Check sheet for the drawn part. Datum: minimum x, y, z corner. Units: mm. Round coordinates to 2 decimals unless told otherwise and drop trailing zeros. Write each loop counter-clockwise with the first axis right and the second up, starting at its lowest first coordinate (ties: lowest second). Pieces come first, ordered by that corner, then holes. Notation, with made-up numbers: (70.5, -4) -> (86.5, -4) arc R6 ccw to (86.5, 6) -> close; hole circle Ø10 at (67, 76.25). An arc over 180 degrees is marked (long way). Use a Markdown table: item, result.
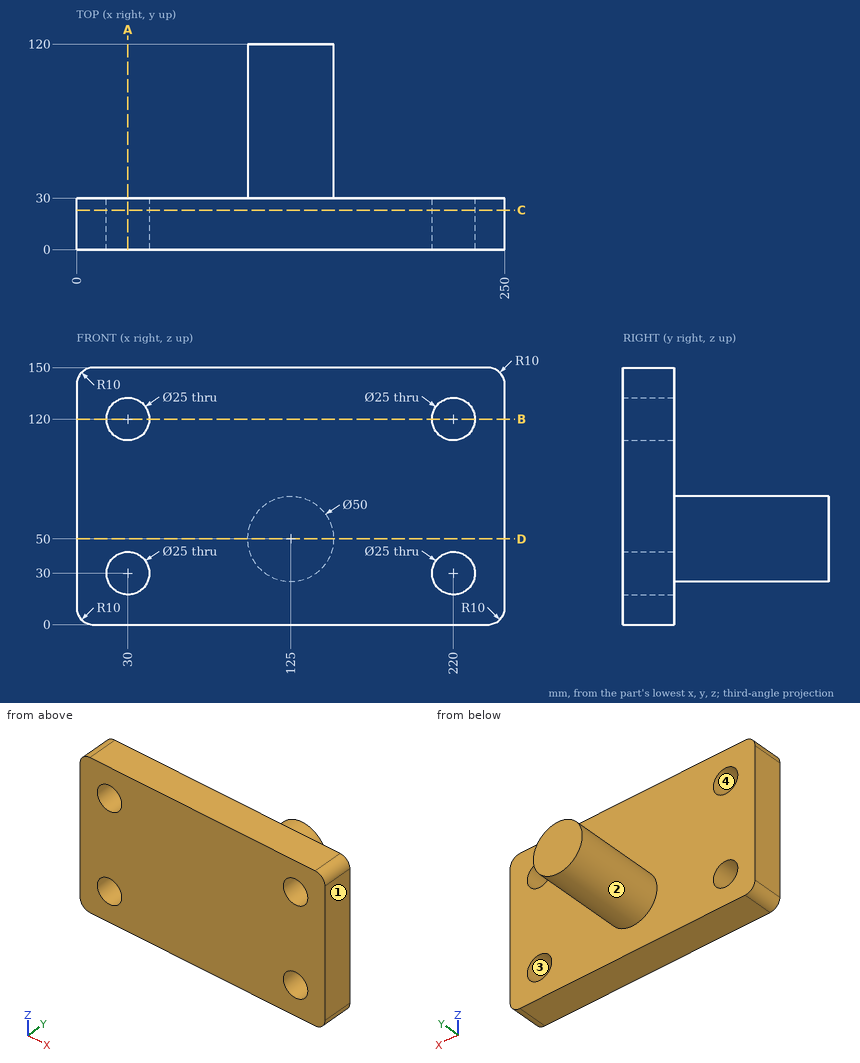
(1) Thickness scan on line 1 (X direction, y = 18, z = 120); line 2 (Z direction, x = 30, y = 19); line 3 (Y direction, x = 207.5, z = 82.5). Record the ranges inside material, lowest first.
A:
| item | result |
|---|---|
| line 1 | x = 0 to 17.5, 42.5 to 207.5, 232.5 to 250 |
| line 2 | z = 0 to 17.5, 42.5 to 107.5, 132.5 to 150 |
| line 3 | y = 0 to 30 |
(2) Section check C-C on y = 23. Record the cut outline in (x, z), plus the area to 3 significant figures.
A:
| item | result |
|---|---|
| outline | (0, 10) arc R10 ccw to (10, 0) -> (240, 0) arc R10 ccw to (250, 10) -> (250, 140) arc R10 ccw to (240, 150) -> (10, 150) arc R10 ccw to (0, 140) -> close; hole circle Ø25 at (30, 30); hole circle Ø25 at (30, 120); hole circle Ø25 at (220, 30); hole circle Ø25 at (220, 120) |
| area | 35,500 mm2 |
(3) Section check A-A on x = 30. Record the cut outline in (y, z), plus the area to 3 significant figures.
A:
| item | result |
|---|---|
| outline | (0, 0) -> (30, 0) -> (30, 17.5) -> (0, 17.5) -> close; (0, 42.5) -> (30, 42.5) -> (30, 107.5) -> (0, 107.5) -> close; (0, 132.5) -> (30, 132.5) -> (30, 150) -> (0, 150) -> close |
| area | 3,000 mm2 |
(4) Section check B-B on z = 120. Record the cut outline in (x, y).
A:
| item | result |
|---|---|
| outline | (0, 0) -> (17.5, 0) -> (17.5, 30) -> (0, 30) -> close; (42.5, 0) -> (207.5, 0) -> (207.5, 30) -> (42.5, 30) -> close; (232.5, 0) -> (250, 0) -> (250, 30) -> (232.5, 30) -> close |
(5) Section check D-D on z = 50. Record the cut outline in (x, y).
A:
| item | result |
|---|---|
| outline | (0, 0) -> (250, 0) -> (250, 30) -> (150, 30) -> (150, 120) -> (100, 120) -> (100, 30) -> (0, 30) -> close |
(6) Gauge pin test, flat ends, axial feed: pin 1 Ø20 at (x, z) = (220, 30) entering from -Y; pin 2 Ø10 at (x, z) = (151, 115.5) entering from +Y; pin 3 Ø3 at (x, y) = (111, 83) entering from +Z; pin 4 Ø5 at (x, y) = (121, 46) entering from +Z. Record the tip position at first contact, or that the pin passes through.
A:
| item | result |
|---|---|
| pin 1 | passes through |
| pin 2 | stops at y = 30 |
| pin 3 | stops at z = 71.65 |
| pin 4 | stops at z = 74.95 |
(7) Release check for a two-part mould opening along X. For the marked faces 1, 2, 3 and 4 record: +X half, -X half, draft (parallel to the pull), parting line (faces both ways), or undercut.
A:
| item | result |
|---|---|
| face 1 | +X half |
| face 2 | parting line |
| face 3 | undercut |
| face 4 | undercut |
